from build123d import *

# Parameters (mm, degrees)
BOSS_EXTRU_1_DEPTH   = 25
D_GAGEMENT_M61_D     = 6.6
D_GAGEMENT_M61_DEPTH = 18.5
TROU_TARAUD_M61_D    = 5
TROU_TARAUD_M41_D    = 3.3
D_GAGEMENT_M81_D     = 9


with BuildPart() as part:
    # Esquisse1 → Boss.-Extru.1 (new body)
    with BuildSketch(Plane(origin=(0, 0, 0), x_dir=(1, 0, 0), z_dir=(0, 1, 0))):
        with BuildLine():
            Line((-87, -1.5), (-87, -20))
            Line((-87, -20), (87, -20))
            Line((87, -20), (87, -1.5))
            Line((87, -1.5), (75.139649895, -1.5))
            ThreePointArc((75.139649895, -1.5), (54.75, 0), (75.139649895, 1.5))
            Line((75.139649895, 1.5), (87, 1.5))
            Line((87, 1.5), (87, 20))
            Line((87, 20), (-87, 20))
            Line((-87, 20), (-87, 1.5))
            Line((-87, 1.5), (-75.176050211, 1.5))
            ThreePointArc((-75.176050211, 1.5), (-59.249089125, 15.231501333), (-44.75, 0))
            ThreePointArc((-44.75, 0), (-59.249089125, -15.231501333), (-75.176050211, -1.5))
            Line((-75.176050211, -1.5), (-87, -1.5))
        make_face()
    extrude(amount=BOSS_EXTRU_1_DEPTH)

    # Dégagement M61
    with Locations(Plane(origin=(80, 12.5, 20), x_dir=(1, 0, 0), z_dir=(0, 0, 1))):
        with Locations((0, 0), (-160, 0)):
            Hole(D_GAGEMENT_M61_D / 2, depth=D_GAGEMENT_M61_DEPTH)

    # Trou taraudé M61 (through all)
    with Locations(Plane(origin=(80, 12.5, -1.5), x_dir=(1, 0, 0), z_dir=(0, 0, 1))):
        with Locations((0, 0), (-160, 0)):
            Hole(TROU_TARAUD_M61_D / 2)

    # Trou taraudé M41 (through all)
    with Locations(Plane(origin=(65, 12.5, 20), x_dir=(1, 0, 0), z_dir=(0, 0, 1))):
        with Locations((0, 0)):
            Hole(TROU_TARAUD_M41_D / 2)

    # Dégagement M81 (through all)
    with Locations(Plane(origin=(0, 25, -11), x_dir=(0, 0, 1), z_dir=(0, 1, 0))):
        with Locations((0, 0), (22, 0)):
            Hole(D_GAGEMENT_M81_D / 2)


solid = part.part
Source: CAD feature listing. Evaluate the final solid. Frame: model axes, mm. A direction names the side the tool comes from. Give positions to 0.01 mm unless a question says otherwise; leave off trailing zeros. Write each loop counter-clockwise with the first axis right and the second up, starting at its lowest first coordinate (ties: lowest second). Pieces come first, ordered by that corner, then holes. Notation, with made-up numbers: (84, -26) -> (101, -26) arc R17 cw to (101, 2) -> close; hole circle Ø11 at (-9, -13). An arc over 180 degrees is marked (long way). Return JSON: item names as keys, results as strings. Group by question number.
1. Material intervals for line 1 (Y direction, x = 65, z = -15); line 2 (Y direction, x = -80, z = -10); line 3 (X direction, y = 8.5, z = -3), sorted ascending. Write a range as from..to.
2. Pin query (flat end, axial travel): pin 1 Ø5.5 at (x, y) = (80, 12.5) entering from +Z. Return the tip coordinate at first contact, or that it passes through.
3. Mould query, pull axis Y, two halves, no side actions, for faces 1 (the face through (-1, 0, 0)), 2 (the face through (-1, 25, 0)), 3 (the face through (-78, 11, -11)), 4 (the face through (-87, 12, 11)). Classes: +Y half, -Y half, draft (parallel to the pull), parting line (faces both ways), or undercut.
4. Section D-D, the plane x = -60. Output: boundary loops of the cut face in (y, z).
5. Section B-B, the plane x = 0. Output: boundary loops of the cut face in (y, z), then the cut area to 3 significant figures.
6. Section C-C, the plane y = 20. Output: boundary loops of the cut face in (x, z).
7. Access query for faces 5 (the face through (84, 12, -1.5)), 6 (the face through (66.31, 11.5, -15.13)), 7 (the face through (-84, 12, 1.5)), 8 (the face through (-76.7, 12.6, 10.6)), 9 (the face through (1.352, 12.325, -15.292)). Directions: +Z, -Z, +X, -X, +Y, -Y. A direction counts if a zero-diameter tool reaches every point of the face in a straight line with its end or side. Return the directions, or none.
8. Section A-A, the plane z = 4. Output: boundary loops of the cut face in (x, y), then the cut area to 3 significant figures.
Determined:
{
 "1": {"line 1": "y = 0..10.85, 14.15..25", "line 2": "y = 0..10, 15..25", "line 3": "x = -87..-74.95, -45.05..55.2, 74.8..87"},
 "2": {"pin 1": "stops at z = -1.5"},
 "3": {"face 1": "-Y half", "face 2": "+Y half", "face 3": "undercut", "face 4": "draft"},
 "4": {"outline": "(0, -20) -> (25, -20) -> (25, -15.25) -> (0, -15.25) -> close; (0, 15.25) -> (25, 15.25) -> (25, 20) -> (0, 20) -> close"},
 "5": {"outline": "(0, -20) -> (25, -20) -> (25, -15.5) -> (0, -15.5) -> close; (0, -6.5) -> (25, -6.5) -> (25, 6.5) -> (0, 6.5) -> close; (0, 15.5) -> (25, 15.5) -> (25, 20) -> (0, 20) -> close", "area": "550 mm2"},
 "6": {"outline": "(-87, -20) -> (87, -20) -> (87, -1.5) -> (75.14, -1.5) arc R10.25 cw (long way) to (75.14, 1.5) -> (87, 1.5) -> (87, 20) -> (-87, 20) -> (-87, 1.5) -> (-75.18, 1.5) arc R15.25 cw (long way) to (-75.18, -1.5) -> (-87, -1.5) -> close; hole circle Ø9 at (0, -11); hole circle Ø9 at (0, 11)"},
 "7": {"face 5": "+X, +Y, -Y", "face 6": "+Z, -Z", "face 7": "-X, +Y, -Y", "face 8": "+Z", "face 9": "+Y, -Y"},
 "8": {"outline": "(-87, 0) -> (-74.72, 0) -> (-74.72, 25) -> (-87, 25) -> close; (-45.28, 0) -> (55.56, 0) -> (55.56, 25) -> (-45.28, 25) -> close; (74.44, 0) -> (87, 0) -> (87, 25) -> (74.44, 25) -> close; hole circle Ø6.6 at (-80, 12.5); hole circle Ø6.6 at (80, 12.5)", "area": "3,070 mm2"}
}
